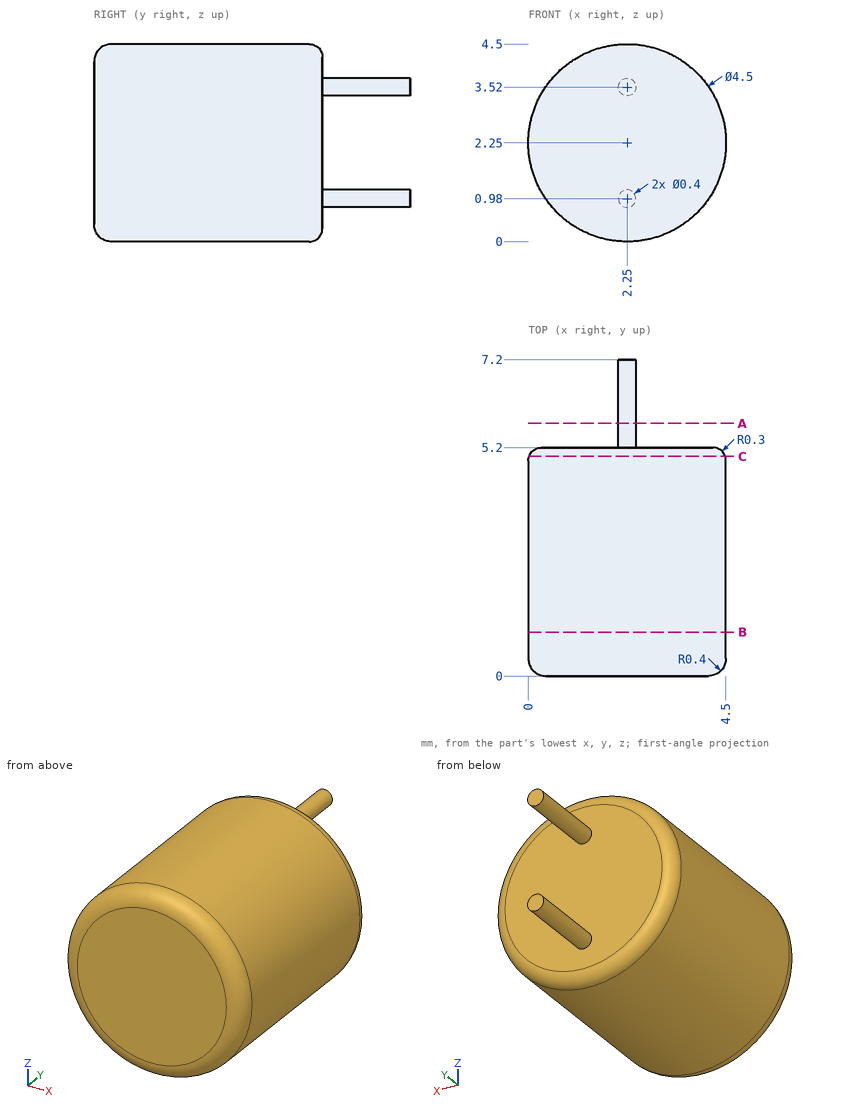
Geometry check sheet. Reference: drawing and pictorial views, mm from the part's lowest x, y, z. Coordinates: 2 decimals unless noted, no trailing zeros. Loops run counter-clockwise (first coordinate to the right, second up) from the corner with the lowest first, then second, coordinate; pieces in that order, holes last.
1) Material ranges on probe 1 along Y at (x, z) = (2.55, 1.55); probe 2 along X at (y, z) = (0.5, 3.1); probe 3 along X at (y, z) = (4.75, 3), recorded low to high.
2) Sectioned sample at B-B (y = 1). Record the boundary of the cut face in (x, z).
3) Gauge pin test, flat ends, axial feed: pin 1 (1 mm diameter, centred on x = 1.5, y = 2, fed in from +Z); pin 2 (1 mm diameter, centred on y = 5.5, z = 1, fed in from +X); pin 3 (1 mm diameter, centred on y = 1.5, z = 0.5, fed in from +X). Record the tip position at first contact, or that the pin passes through.
4) Sectioned sample at C-C (y = 5). Record the boundary of the cut face in (x, z).
5) Sectioned sample at A-A (y = 5.75). Record the boundary of the cut face in (x, z), and give its area (3 significant figures).
Check sheet entries:
1. probe 1: y = 0 to 5.2
1. probe 2: x = 0.17 to 4.33
1. probe 3: x = 0.13 to 4.37
2. outline: circle Ø4.5 at (2.25, 2.25)
3. pin 1: stops at z = 4.49
3. pin 2: stops at x = 4.21
3. pin 3: stops at x = 4.12
4. outline: circle Ø4.47 at (2.25, 2.25)
5. outline: circle Ø0.4 at (2.25, 0.98); circle Ø0.4 at (2.25, 3.52)
5. area: 0.251 mm2
